Input: part model. Units: mm. Frame: model coordinates. Coordinates: 2 decimals unless noted, no trailing zeros. Order: outer loops, then holes, each group sorted by start corner. A loop starts at its lowest first (then second) coordinate and runs counter-clockwise, first axis right, second up. Notation, with made-up numbers: M 59,-14 L 79,-14 A29 ccw 79,19 Z; hole C 79.25,-14.5 d10. An arc over 180 degrees is marked long. Answer in a Markdown table with one row per item.
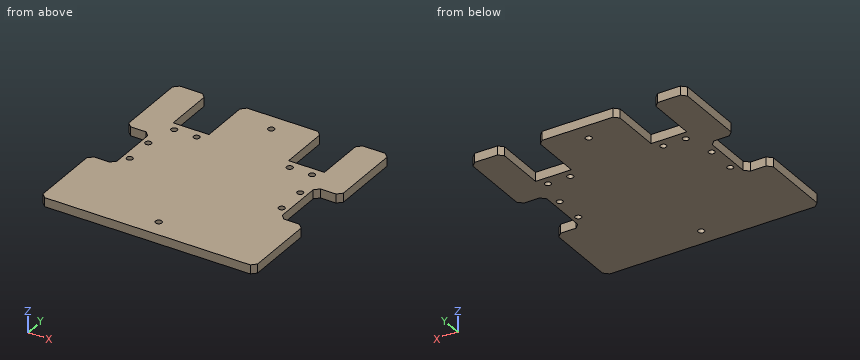
Autodesk Inventor part; units mm, degrees
ref_plane "YZ Plane" through (0, 0, 0) normal (1, 0, 0) x (0, 1, 0)
ref_plane "XZ Plane" through (0, 0, 0) normal (0, 1, 0) x (-1, 0, 0)
ref_plane "XY Plane" through (0, 0, 0) normal (0, 0, 1) x (1, 0, 0)
sketch "Sketch1" plane through (0, 0, 0) normal (0, 0, 1) x (1, 0, 0)
  line L0 (0, 0) -> (152.4, 0)
  line L1 (152.4, 96.8375) -> (134.9375, 96.8375)
  line L2 (134.9375, 96.8375) -> (134.9375, 55.5625)
  line L3 (134.9375, 55.5625) -> (152.4, 55.5625)
  line L4 (0, 96.8375) -> (17.4625, 96.8375)
  line L5 (17.4625, 96.8375) -> (17.4625, 55.5625)
  line L6 (17.4625, 55.5625) -> (0, 55.5625)
  line L7 (152.4, 0) -> (152.4, 55.5625)
  line L8 (152.4, 96.8375) -> (152.4, 152.4)
  line L9 (0, 152.4) -> (0, 96.8375)
  line L10 (0, 55.5625) -> (0, 0)
  circle A0 centre (22.225, 86.6775) radius 2.1526
  circle A1 centre (22.225, 65.7225) radius 2.1526
  circle A2 centre (130.175, 86.6775) radius 2.1526
  circle A3 centre (130.175, 65.7225) radius 2.1526
  line L11 (22.479, 152.4) -> (22.479, 114.3)
  line L12 (22.479, 114.3) -> (47.879, 114.3)
  line L13 (47.879, 114.3) -> (47.879, 152.4)
  line L14 (104.521, 152.4) -> (104.521, 114.3)
  line L15 (104.521, 114.3) -> (129.921, 114.3)
  line L16 (129.921, 114.3) -> (129.921, 152.4)
  line L17 (22.479, 152.4) -> (0, 152.4)
  line L18 (152.4, 152.4) -> (129.921, 152.4)
  line L19 (104.521, 152.4) -> (47.879, 152.4)
  dimension "d0" = 152.4
  dimension "d1" = 152.4
  dimension "d2" = 41.275
  dimension "d3" = 55.5625
  dimension "d4" = 17.4625
  dimension "d5" = 41.275
  dimension "d6" = 17.4625
  dimension "d7" = 55.5625
  dimension "d8" = 152.4
  dimension "d10" = 4.3053
  dimension "d11" = 4.3053
  dimension "d12" = 4.3053
  dimension "d13" = 4.3053
  dimension "d15" = 22.225
  dimension "d16" = 22.225
  dimension "d17" = 22.225
  dimension "d18" = 22.225
  dimension "d19" = 10.16
  dimension "d20" = 10.16
  dimension "d21" = 10.16
  dimension "d22" = 10.16
  dimension "d28" = 107.442
  dimension "d29" = 25.4
  dimension "d30" = 25.4
  dimension "d31" = 22.479
  dimension "d32" = 38.1
extrude "Extrusion1" add sketch "Sketch1" along normal blind 6.35
chamfer "Chamfer1" distance 3.175 angle 45 12 edges at (0, 55.5625, 3.175) (17.4625, 55.5625, 3.175) (17.4625, 96.8375, 3.175) (0, 96.8375, 3.175) (152.4, 55.5625, 3.175) (134.9375, 55.5625, 3.175) (134.9375, 96.8375, 3.175) (152.4, 96.8375, 3.175) (152.4, 0, 3.175) (0, 0, 3.175) (0, 152.4, 3.175) (152.4, 152.4, 3.175)
chamfer "Chamfer2" distance 3.175 angle 45 4 edges at (22.479, 152.4, 3.175) (47.879, 152.4, 3.175) (104.521, 152.4, 3.175) (129.921, 152.4, 3.175)
sketch "Sketch2" plane through (0, 0, 0) normal (0, 0, -1) x (-1, 0, 0)
  line L0 (-22.479, 114.3) -> (-22.479, 149.225)
  line L1 (-129.921, 114.3) -> (-104.521, 114.3)
  line L2 (-129.921, 149.225) -> (-129.921, 114.3)
  line L3 (-125.1585, 107.95) -> (-27.2415, 107.95) construction
  point P0 (0, 0)
  point P1 (-109.2835, 107.95)
  point P2 (-43.1165, 107.95)
  dimension "d37" = 15.875
  dimension "d39" = 15.875
  dimension "d40" = 4.7625
  dimension "d41" = 4.7625
  dimension "d42" = 6.35
hole "Hole1" at (109.2835, 107.95, 0) at (43.1165, 107.95, 0) at (27.2415, 107.95, 0) at (125.1585, 107.95, 0) direction (0, 0, 1) diameter 4.3053 end through all
sketch "Sketch3" plane through (0, 0, 6.35) normal (0, 0, 1) x (1, 0, 0)
  line L0 (101.346, 152.4) -> (51.054, 152.4)
  line L1 (3.175, 0) -> (149.225, 0)
  point P0 (0, 0)
  point P1 (76.2, 139.7)
  point P2 (76.2, 12.7)
  dimension "d50" = 76.2
  dimension "d51" = 76.2
  dimension "d52" = 12.7
  dimension "d53" = 12.7
hole "Hole2" at (76.2, 139.7, 6.35) at (76.2, 12.7, 6.35) direction (0, 0, -1) diameter 4.4958 end through all
equation "\"d31\" = -0.5 * d28 + 0.5 * d0"
properties part number "base"
1) Material intervals for probe 1 along X at (y, z) = (117, 5); probe 2 along Y at (x, z) = (76.2, 2.5); probe 3 along X at (y, z) = (87.5, 2.25), sorted ascending.
Resolved:
| item | result |
|---|---|
| probe 1 | x = 0 to 22.48, 47.88 to 104.52, 129.92 to 152.4 |
| probe 2 | y = 0 to 10.45, 14.95 to 137.45, 141.95 to 152.4 |
| probe 3 | x = 17.46 to 20.24, 24.21 to 128.19, 132.16 to 134.94 |
2) Cut plane C-C, the plane x = 76.2. Output: boundary loops of the cut face in (y, z).
Resolved:
| item | result |
|---|---|
| outline | M 0,0 L 10.45,0 L 10.45,6.35 L 0,6.35 Z; M 14.95,0 L 137.45,0 L 137.45,6.35 L 14.95,6.35 Z; M 141.95,0 L 152.4,0 L 152.4,6.35 L 141.95,6.35 Z |
3) Cut plane D-D, the plane y = 12.7. Output: boundary loops of the cut face in (x, z).
Resolved:
| item | result |
|---|---|
| outline | M 0,0 L 73.95,0 L 73.95,6.35 L 0,6.35 Z; M 78.45,0 L 152.4,0 L 152.4,6.35 L 78.45,6.35 Z |
4) Cut plane B-B, the plane y = 139.7. Output: boundary loops of the cut face in (x, z), and give its area (3 significant figures).
Resolved:
| item | result |
|---|---|
| outline | M 0,0 L 22.48,0 L 22.48,6.35 L 0,6.35 Z; M 47.88,0 L 73.95,0 L 73.95,6.35 L 47.88,6.35 Z; M 78.45,0 L 104.52,0 L 104.52,6.35 L 78.45,6.35 Z; M 129.92,0 L 152.4,0 L 152.4,6.35 L 129.92,6.35 Z |
| area | 617 mm2 |
5) Cut plane A-A, the plane y = 107.95. Output: boundary loops of the cut face in (x, z).
Resolved:
| item | result |
|---|---|
| outline | M 0,0 L 25.09,0 L 25.09,6.35 L 0,6.35 Z; M 29.39,0 L 40.96,0 L 40.96,6.35 L 29.39,6.35 Z; M 45.27,0 L 107.13,0 L 107.13,6.35 L 45.27,6.35 Z; M 111.44,0 L 123.01,0 L 123.01,6.35 L 111.44,6.35 Z; M 127.31,0 L 152.4,0 L 152.4,6.35 L 127.31,6.35 Z |
6) Contact query for flat-ended pins moving along their axis: pin 1 (4 mm diameter, centred on x = 22.22, y = 86.68, fed in from -Z); pin 2 (1.9 mm diameter, centred on y = 80, z = 2.5, fed in from +X); pin 3 (1.9 mm diameter, centred on x = 39, z = 2.5, fed in from +Y); pin 4 (1.9 mm diameter, centred on y = 79, z = 2.5, fed in from -X). Output: stop coordinate, or through.
Resolved:
| item | result |
|---|---|
| pin 1 | passes through |
| pin 2 | stops at x = 134.94 |
| pin 3 | stops at y = 114.3 |
| pin 4 | stops at x = 17.46 |
